```python
from build123d import *

# Parameters (mm, degrees)
SKETCH_1_W          = 15
SKETCH_1_H          = 20
EXTRUDE_1_DEPTH     = 25
SKETCH_2_W          = 15
SKETCH_2_H          = 11.5
CUT_EXTRUDE_1_DEPTH = 5
SKETCH_3_R          = 1.5
CUT_EXTRUDE_2_DEPTH = 24.58495283
SKETCH_4_R          = 1.25
CUT_EXTRUDE_3_DEPTH = 33.882366095
CHAMFER_1_SIZE      = 1
SKETCH_5_W          = 15
SKETCH_5_H          = 7
CUT_EXTRUDE_4_DEPTH = 3.5


with BuildPart() as part:
    # 草图1 → 凸台-拉伸1 (new body)
    with BuildSketch(Plane(origin=(0, 0, 0), x_dir=(0, 0, -1), z_dir=(1, 0, 0))):
        Rectangle(SKETCH_1_W, SKETCH_1_H)
    extrude(amount=EXTRUDE_1_DEPTH)

    # 草图2 → 切除-拉伸1 (cut)
    with BuildSketch(Plane.ZY):
        Rectangle(SKETCH_2_W, SKETCH_2_H)
    extrude(amount=-CUT_EXTRUDE_1_DEPTH, mode=Mode.SUBTRACT)

    # 草图3 → 切除-拉伸2 (cut, through all)
    with BuildSketch(Plane.ZY.offset(-5)):
        with Locations((-4.25, 0)):
            Circle(SKETCH_3_R)
        with Locations((4.25, 0)):
            Circle(SKETCH_3_R)
    extrude(amount=-CUT_EXTRUDE_2_DEPTH, mode=Mode.SUBTRACT)

    # 草图4 → 切除-拉伸3 (cut, through all)
    with BuildSketch(Plane(origin=(0, 10, 0), x_dir=(1, 0, 0), z_dir=(0, 1, 0))):
        with Locations(Location((20, 0, 0), (0, 0, 270))):
            Circle(SKETCH_4_R)
        with Locations(Location((10, 0, 0), (0, 0, 270))):
            Circle(SKETCH_4_R)
    extrude(amount=-CUT_EXTRUDE_3_DEPTH, mode=Mode.SUBTRACT)

    # 倒角1
    chamfer_1_edges = [part.edges().sort_by_distance(p)[0] for p in [
        (12.5, 10, 7.5),
        (12.5, 10, -7.5),
        (12.5, -10, -7.5),
        (12.5, -10, 7.5),
    ]]
    chamfer(chamfer_1_edges, length=CHAMFER_1_SIZE)

    # 草图5 → 切除-拉伸4 (cut)
    with BuildSketch(Plane(origin=(25, 0, 0), x_dir=(0, 0, -1), z_dir=(1, 0, 0))):
        Rectangle(SKETCH_5_W, SKETCH_5_H)
    extrude(amount=-CUT_EXTRUDE_4_DEPTH, mode=Mode.SUBTRACT)


solid = part.part
```
Can you work these out from the model? Positions are in its coordinate system, mm. A direction names the side the tool comes from. Coordinates: 2 decimals unless noted, no trailing zeros. Order: outer loops, then holes, each group sorted by start corner. A loop starts at its lowest first (then second) coordinate and runs counter-clockwise, first axis right, second up.
1. I'm going to push flat-ended pins straight in: pin 1 (1 mm diameter, centred on y = 1.5, z = -6, fed in from -X); pin 2 (2 mm diameter, centred on y = 0, z = 1.5, fed in from +X); pin 3 (2 mm diameter, centred on x = 10, z = 0, fed in from -Y). Where does each tip first touch, or does it pass through?
2. If we section it at D-D (y = -5.25): Please give me the cut outline in (x, z).
3. For faces 4 (the face through (2, 5.75, 0)), 5 (the face through (12.3, -9.5, 7)), 6 (the face through (23, -3.5, 0)), which set-ups out of +Z, -Z, +X, -X, +Y, -Y let a thin tool reach every point of the face, with its end or its side?
4. If we section it at B-B (z = -4.25): Please give me the cut outline in (x, y), then the cut area to 4 significant figures.
5. If we section it at A-A (x = 20): Please give me the cut outline in (y, z), then the cut area to 3 significant figures.
6. Thinking about a two-plate mould opening in Y: for faces 1 (the face through (5, 0, 0)), 2 (the face through (12, 0, 7.5)), 3 (the face through (12, -10, 0)), which applies, +Y half, -Y half, draft (parallel to the pull), parting line (faces both ways), or undercut?
7. If we section it at C-C (y = 0): Please give me the cut outline in (x, z), then the cut area to 3 significant figures.
8. I need wall thicknesses on line 1 (X direction, y = 4.25, z = 0); line 2 (X direction, y = 0.25, z = 0); line 3 (Y direction, x = 22, z = -0.5). Which ranges of each line are inside material? Lowest first, please.
Entries:
1. pin 1: stops at x = 5
1. pin 2: stops at x = 21.5
1. pin 3: passes through
2. outline: (5, -7.5) - (25, -7.5) - (25, 7.5) - (5, 7.5) - close; hole circle Ø2.5 at (10, 0); hole circle Ø2.5 at (20, 0)
3. face 4: +Z, -Z, -X
3. face 5: +Z, +X, -X, -Y
3. face 6: +Z, -Z, +X
4. outline: (0, -10) - (25, -10) - (25, -3.5) - (21.5, -3.5) - (21.5, -1.5) - (5, -1.5) - (5, -5.75) - (0, -5.75) - close; (0, 5.75) - (5, 5.75) - (5, 1.5) - (21.5, 1.5) - (21.5, 3.5) - (25, 3.5) - (25, 10) - (0, 10) - close
4. area: 368.5 mm2
5. outline: (-10, -6.5) - (-9, -7.5) - (9, -7.5) - (10, -6.5) - (10, -1.25) - (-10, -1.25) - close; (-10, 1.25) - (10, 1.25) - (10, 6.5) - (9, 7.5) - (-9, 7.5) - (-10, 6.5) - close; hole circle Ø3 at (0, -4.25); hole circle Ø3 at (0, 4.25)
5. area: 234 mm2
6. face 1: undercut
6. face 2: draft
6. face 3: -Y half
7. outline: (5, -7.5) - (21.5, -7.5) - (21.5, -5.75) - (5, -5.75) - close; (5, -2.75) - (21.5, -2.75) - (21.5, 2.75) - (5, 2.75) - close; (5, 5.75) - (21.5, 5.75) - (21.5, 7.5) - (5, 7.5) - close; hole circle Ø2.5 at (10, 0); hole circle Ø2.5 at (20, 0)
7. area: 139 mm2
8. line 1: x = 5 to 8.75, 11.25 to 18.75, 21.25 to 25
8. line 2: x = 5 to 8.75, 11.25 to 18.75, 21.25 to 21.5
8. line 3: y = -10 to -3.5, 3.5 to 10
